Drawing for the job (mm, zero at the part's lowest x, y, z). Round coordinates to 2 decimals unless told otherwise and drop trailing zeros. Write each loop counter-clockwise with the first axis right and the second up, starting at its lowest first coordinate (ties: lowest second). Pieces come first, ordered by that corner, then holes. Notation, with made-up numbers: (41, 38) - (53, 38) arc R15 cw to (53, 46) - close; hole circle Ø8 at (70, 25). An arc over 180 degrees is marked (long way). One line per question, with ' | ' between items.
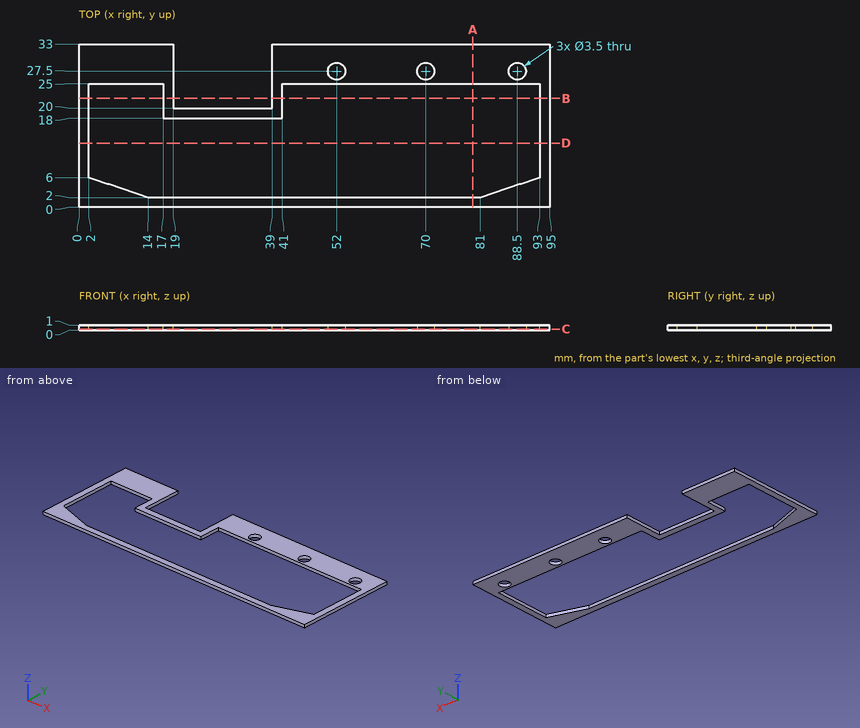
Q1. Drop a flat-ended pin along its axis: pin 1 (0.5 mm diameter, centred on x = 27, z = 0.5, fed in from +Y). Give the stop position or say it passes through.
Found:
pin 1: y = 20
Q2. Saw through at B-B, the plane y = 22. List the corners of the cut face in (x, z).
Found:
outline: (0, 0) - (2, 0) - (2, 1) - (0, 1) - close; (17, 0) - (19, 0) - (19, 1) - (17, 1) - close; (39, 0) - (41, 0) - (41, 1) - (39, 1) - close; (93, 0) - (95, 0) - (95, 1) - (93, 1) - close
Q3. Drill centre lines: L1, parallel to Y at x = 70, z = 0.7; L2, parallel to X at y = 21, z = 0.2; L3, parallel to X at y = 19.5, z = 0.7. Where is each one in solid material? Low to high. Write a range as from..to.
Found:
L1: 0..2, 25..25.75, 29.25..33 | L2: 0..2, 17..19, 39..41, 93..95 | L3: 0..2, 17..41, 93..95
Q4. Saw through at D-D, the plane y = 13. List the corners of the cut face in (x, z).
Found:
outline: (0, 0) - (2, 0) - (2, 1) - (0, 1) - close; (93, 0) - (95, 0) - (95, 1) - (93, 1) - close
Q5. Saw through at C-C, the plane z = 0.25. List the corners of the cut face in (x, y), then the cut area to 3 significant figures.
Found:
outline: (0, 0) - (95, 0) - (95, 33) - (39, 33) - (39, 20) - (19, 20) - (19, 33) - (0, 33) - close; hole (2, 6) - (14, 2) - (81, 2) - (93, 6) - (93, 25) - (41, 25) - (41, 18) - (17, 18) - (17, 25) - (2, 25) - close; hole circle Ø3.5 at (52, 27.5); hole circle Ø3.5 at (70, 27.5); hole circle Ø3.5 at (88.5, 27.5) | area: 969 mm^2
Q6. Saw through at A-A, the plane x = 79.5. List the corners of the cut face in (y, z), then the cut area to 3 significant figures.
Found:
outline: (0, 0) - (2, 0) - (2, 1) - (0, 1) - close; (25, 0) - (33, 0) - (33, 1) - (25, 1) - close | area: 10.0 mm^2
